Can you work these out from the drawing? Everything is in mm from the part's minimum corner. Coordinates: 2 decimals unless noted, no trailing zeros. Order: outer loops, then holes, each group sorted by start corner. A loop starts at its lowest first (then second) coordinate and runs counter-clockwise, first axis right, second up. Notation, with made-up numbers: (6, -0.5) - (17, -0.5) arc R13 ccw to (17, 20.5) - close; hole circle Ø1 at (-1.75, 38). An arc over 180 degrees is marked (long way). Answer as CSV lines item,"result". Start each with the question number.
Q1. Suppose I cut it at A-A (y = 6.35). Please give me the cut outline in (x, z), then the cut area to 3 significant figures.
Q2. I need wall thicknesses on line 1 (X direction, y = 4.25, z = 0.1); line 2 (X direction, y = 5.5, z = 0.2); line 3 (Y direction, x = 9.5, z = 0.1). Which ranges of each line are inside material? Lowest first, please.
Q3. Suppose I cut it at C-C (z = 0.15). Please give me the cut outline in (x, y) (3 decimals), then the cut area to 3 significant figures.
Q4. Suppose I cut it at B-B (x = 7.5). Please give me the cut outline in (y, z), then the cut area to 3 significant figures.
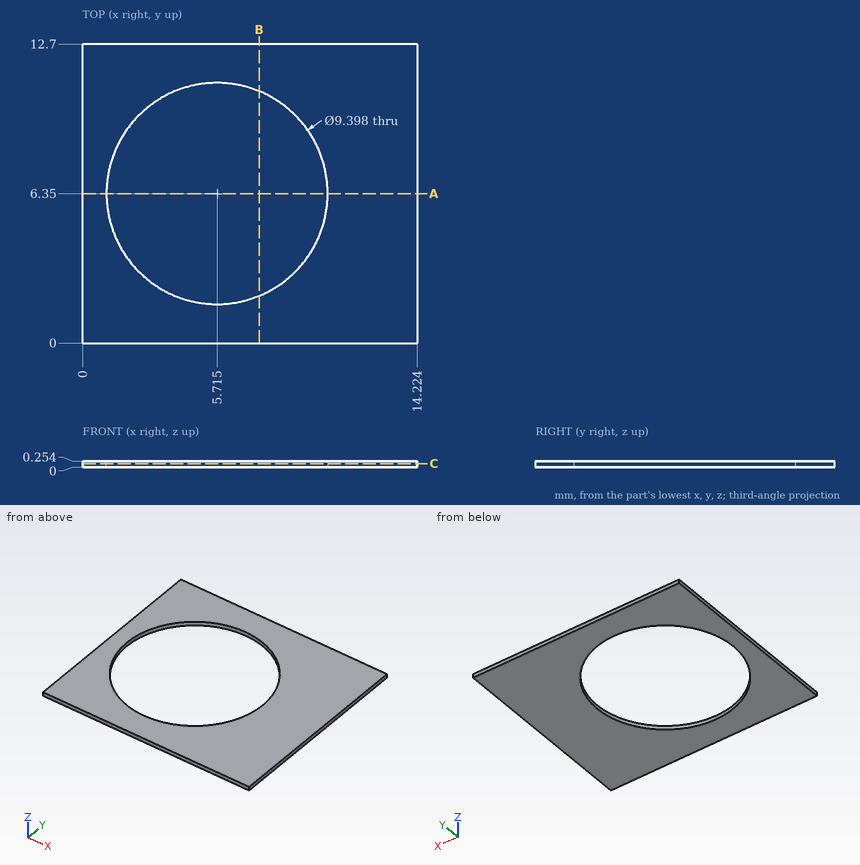
Here are the results:
1,outline,"(0, 0) - (1.02, 0) - (1.02, 0.25) - (0, 0.25) - close; (10.41, 0) - (14.22, 0) - (14.22, 0.25) - (10.41, 0.25) - close"
1,area,"1.23 mm²"
2,line 1,"x = 0 to 1.51, 9.92 to 14.22"
2,line 2,"x = 0 to 1.09, 10.34 to 14.22"
2,line 3,"y = 0 to 3.57, 9.13 to 12.7"
3,outline,"(0, 0) - (14.224, 0) - (14.224, 12.7) - (0, 12.7) - close; hole circle Ø9.398 at (5.715, 6.35)"
3,area,"111 mm²"
4,outline,"(0, 0) - (2, 0) - (2, 0.25) - (0, 0.25) - close; (10.7, 0) - (12.7, 0) - (12.7, 0.25) - (10.7, 0.25) - close"
4,area,"1.02 mm²"
